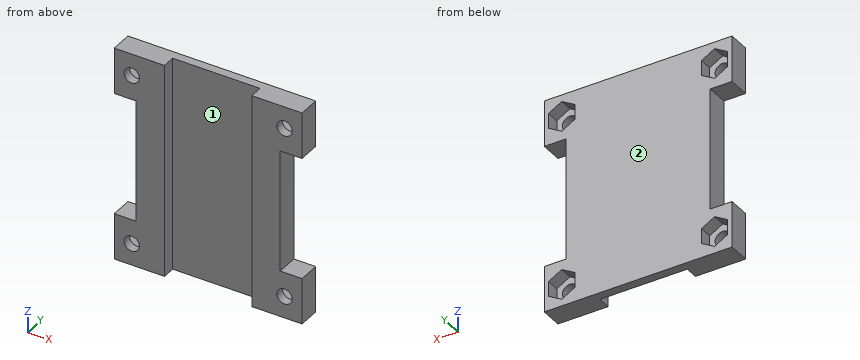
from build123d import *

# Parameters (mm, degrees)
SKETCH1_W           = 43
SKETCH1_H           = 49.17
BOSS_EXTRUDE1_DEPTH = 5
CUT_EXTRUDE1_DEPTH  = 3
SKETCH4_R           = 1.75
CUT_EXTRUDE2_DEPTH  = 66.388752091
SKETCH5_W           = 5
SKETCH5_H           = 28
CUT_EXTRUDE3_DEPTH  = 66.510983049
SKETCH7_W           = 20
SKETCH7_H           = 49.17
CUT_EXTRUDE4_DEPTH  = 3


with BuildPart() as part:
    # Sketch1 → Boss-Extrude1 (new body)
    with BuildSketch(Plane(origin=(0, 0, 0), x_dir=(1, 0, 0), z_dir=(0, 1, 0))):
        with Locations((-21.5, 24.585)):
            Rectangle(SKETCH1_W, SKETCH1_H)
    extrude(amount=BOSS_EXTRUDE1_DEPTH)

    # Sketch2 → Cut-Extrude1 (cut)
    with BuildSketch(Plane(origin=(0, 5, 0), x_dir=(1, 0, 0), z_dir=(0, 1, 0))):
        Polygon((-1, 42.437949192), (-4, 40.705898385), (-7, 42.437949192), (-7, 45.902050808), (-4, 47.634101615), (-1, 45.902050808), align=None)
        Polygon((-4, 8.464101615), (-7, 6.732050808), (-7, 3.267949192), (-4, 1.535898385), (-1, 3.267949192), (-1, 6.732050808), align=None)
        Polygon((-42, 6.732050808), (-39, 8.464101615), (-36, 6.732050808), (-36, 3.267949192), (-39, 1.535898385), (-42, 3.267949192), align=None)
        Polygon((-42, 45.902050808), (-42, 42.437949192), (-39, 40.705898385), (-36, 42.437949192), (-36, 45.902050808), (-39, 47.634101615), align=None)
    extrude(amount=-CUT_EXTRUDE1_DEPTH, mode=Mode.SUBTRACT)

    # Sketch4 → Cut-Extrude2 (cut, through all)
    with BuildSketch(Plane(origin=(0, 2, 0), x_dir=(1, 0, 0), z_dir=(0, 1, 0))):
        with Locations(Location((-39, 44.17, 0), (0, 0, 270))):
            Circle(SKETCH4_R)
        with Locations(Location((-39, 5, 0), (0, 0, 90))):
            Circle(SKETCH4_R)
        with Locations(Location((-4, 5, 0), (0, 0, 270))):
            Circle(SKETCH4_R)
        with Locations(Location((-4, 44.17, 0), (0, 0, 90))):
            Circle(SKETCH4_R)
    extrude(amount=-CUT_EXTRUDE2_DEPTH, mode=Mode.SUBTRACT)

    # Sketch5 → Cut-Extrude3 (cut, through all)
    with BuildSketch(Plane(origin=(0, 5, 0), x_dir=(1, 0, 0), z_dir=(0, 1, 0))):
        with Locations((-2.5, 24.585)):
            Rectangle(SKETCH5_W, SKETCH5_H)
        with Locations((-40.5, 24.585)):
            Rectangle(SKETCH5_W, SKETCH5_H)
    extrude(amount=-CUT_EXTRUDE3_DEPTH, mode=Mode.SUBTRACT)

    # Sketch7 → Cut-Extrude4 (cut)
    with BuildSketch(Plane.XZ):
        with Locations((-21.5, -24.585)):
            Rectangle(SKETCH7_W, SKETCH7_H)
    extrude(amount=-CUT_EXTRUDE4_DEPTH, mode=Mode.SUBTRACT)


solid = part.part
Build history of the part. All positions in model axes, mm. Face numbers are marked on the shaded views. Round coordinates to 2 decimals unless told otherwise and drop trailing zeros. Loops run counter-clockwise (first coordinate to the right, second up) from the corner with the lowest first, then second, coordinate; pieces in that order, holes last. Notation, with made-up numbers: (51.25, 58.5) -> (94.25, 58.5) arc R16 cw to (94.25, 74.5) -> close; hole circle Ø11 at (-40, 32.25). An arc over 180 degrees is marked (long way). Use CSV: the item, a comma, the result in double quotes. Start each with the question number.
Q1. Mould opens along X. For the marked faces 1 and 2 say: +X half, -X half, draft (parallel to the pull), parting line (faces both ways), or undercut.
Q2. Saw through at C-C on z = -25.5. Give the cut face in (x, y), and give its area (3 significant figures).
Q3. Saw through at D-D on x = -28. Give the cut face in (y, z), and give its area (3 significant figures).
Q4. Saw through at A-A on y = 1.2. Give the cut face in (x, z) (3 decimals).
Q5. Flat gauge pin, fed straight in: pin 1 Ø1.5 at (y, z) = (3.5, -30.5) entering from -X. Where does the tip first touch, or does it go through?
Q6. Drill centre lines: L1, parallel to X at y = 0.8, z = -5; L2, parallel to X at y = 1, z = -37.5; L3, parallel to Y at x = -20.5, z = -27. Where is each one in solid material? Low to high.
Q7. Saw through at B-B on z = -5. Give the cut face in (x, y).
Solutions:
1,face 1,"undercut"
1,face 2,"draft"
2,outline,"(-38, 0) -> (-31.5, 0) -> (-31.5, 3) -> (-11.5, 3) -> (-11.5, 0) -> (-5, 0) -> (-5, 5) -> (-38, 5) -> close"
2,area,"105 mm^2"
3,outline,"(3, -49.17) -> (5, -49.17) -> (5, 0) -> (3, 0) -> close"
3,area,"98.3 mm^2"
4,outline,"(-43, -49.17) -> (-31.5, -49.17) -> (-31.5, 0) -> (-43, 0) -> (-43, -10.585) -> (-38, -10.585) -> (-38, -38.585) -> (-43, -38.585) -> close; (-11.5, -49.17) -> (0, -49.17) -> (0, -38.585) -> (-5, -38.585) -> (-5, -10.585) -> (0, -10.585) -> (0, 0) -> (-11.5, 0) -> close; hole circle Ø3.5 at (-39, -44.17); hole circle Ø3.5 at (-39, -5); hole circle Ø3.5 at (-4, -44.17); hole circle Ø3.5 at (-4, -5)"
5,pin 1,"stops at x = -38"
6,L1,"x = -43 to -40.75, -37.25 to -31.5, -11.5 to -5.75, -2.25 to 0"
6,L2,"x = -38 to -31.5, -11.5 to -5"
6,L3,"y = 3 to 5"
7,outline,"(-43, 0) -> (-40.75, 0) -> (-40.75, 2) -> (-42, 2) -> (-42, 5) -> (-43, 5) -> close; (-37.25, 0) -> (-31.5, 0) -> (-31.5, 3) -> (-11.5, 3) -> (-11.5, 0) -> (-5.75, 0) -> (-5.75, 2) -> (-7, 2) -> (-7, 5) -> (-36, 5) -> (-36, 2) -> (-37.25, 2) -> close; (-2.25, 0) -> (0, 0) -> (0, 5) -> (-1, 5) -> (-1, 2) -> (-2.25, 2) -> close"
